Build history of the part. All positions in model axes, mm. A direction names the side the tool comes from. Give positions to 0.01 mm unless a question says otherwise; leave off trailing zeros. Order: outer loops, then holes, each group sorted by start corner. A loop starts at its lowest first (then second) coordinate and runs counter-clockwise, first axis right, second up. Notation, with made-up numbers: M 8,42.25 L 49,42.25 A10 cw 49,47.25 Z; hole C 27.25,-39.5 d7. An arc over 180 degrees is marked long. Use CSV: the item, a comma, the result in double quotes. Start each with the question number.
Item 1: Band-saw the part on C-C on x = 3.5. Write the cut outline in (y, z) (3 decimals).
Item 2: Pin check, flat tips, straight feed: P1, Ø4.5, axis at y = 14.29, z = 14.29, coming from the +X side; P2, Ø4, axis at x = 22, z = -3, coming from the +Y side; P3, Ø4, axis at x = 7.5, y = 14, coming from the -Z side. Stop position of each tip, or through.
Item 3: Band-saw the part on A-A on z = 0. Write the cut outline in (x, y) (1 decimal).
Item 4: Band-saw the part on D-D on x = 24. Write the cut outline in (y, z), plus the area to 3 significant figures.
Item 5: Two-plate mould, pull along Z, no slides. Class faces 4 (the cylindrical face through (11.845, 16.176, 14.04)), 5 (the cylindrical face through (11.85, -17.32, 17.37)), 6 (the flat face through (12, -18.224, 0)): pulls with the +Z half, pulls with the -Z half, needs draft (parallel to the pull), parting line crosses it, or undercut.
Item 6: Wall check: line 1 along X through (y, z) = (-2, 15.5); line 2 along Y through (x, z) = (20.5, -0.5); line 3 along Y through (x, z) = (16.75, 10). Give the ranges that are in metal, low to high.
Item 7: Which spindle directions (+Z, -Z, +X, -X, +Y, -Y) get a long thin tool onto all of the face, cutting with end or side? Do faces 1 (the cylindrical face through (11.85, 17.32, -17.37)), 2 (the flat face through (10.668, -12, 8)), 3 (the cylindrical face through (20.216, -4.158, 13.204)). Say none if no direction does.
from build123d import *

# Parameters (mm, degrees)
SKETCH2_OUTSIDE_W  = 79.82
SKETCH2_OUTSIDE_H  = 79.82
SKETCH2_OUTSIDE_R  = 1.905
CUT_EXTRUDE1_DEPTH = 17.51


with BuildPart() as part:
    # Sketch1 → Revolve1 (revolve)
    with BuildSketch(Plane.XY, mode=Mode.PRIVATE) as revolve1_sk:
        Polygon((0, 0), (0, 13.335), (10.668, 13.335), (10.668, 30), (13.0556, 30), (13.0556, 13.843), (27.178, 13.843), (27.178, 0), align=None)
    revolve(revolve1_sk.sketch.rotate(Axis((0, 0, 0), (1, 0, 0)), 90), axis=Axis((0, 0, 0), (1, 0, 0)))  # turned: the seam where the file's is

    # Sketch2 outside → Cut-Extrude1 (cut, through all)
    with BuildSketch(Plane.ZY.offset(-10.668)):
        Rectangle(SKETCH2_OUTSIDE_W, SKETCH2_OUTSIDE_H)
        with BuildLine():
            Line((-15.2245, 18.2245), (15.2245, 18.2245))
            ThreePointArc((15.2245, 18.2245), (17.345820344, 17.345820344), (18.2245, 15.2245))
            Line((18.2245, 15.2245), (18.2245, -15.2245))
            ThreePointArc((18.2245, -15.2245), (17.345820344, -17.345820344), (15.2245, -18.2245))
            Line((15.2245, -18.2245), (-15.2245, -18.2245))
            ThreePointArc((-15.2245, -18.2245), (-17.345820344, -17.345820344), (-18.2245, -15.2245))
            Line((-18.2245, -15.2245), (-18.2245, 15.2245))
            ThreePointArc((-18.2245, 15.2245), (-17.345820344, 17.345820344), (-15.2245, 18.2245))
        make_face(mode=Mode.SUBTRACT)
        with Locations((14.2875, 14.2875)):
            Circle(SKETCH2_OUTSIDE_R)
        with Locations((-14.2875, 14.2875)):
            Circle(SKETCH2_OUTSIDE_R)
        with Locations((-14.2875, -14.2875)):
            Circle(SKETCH2_OUTSIDE_R)
        with Locations((14.2875, -14.2875)):
            Circle(SKETCH2_OUTSIDE_R)
    extrude(amount=-CUT_EXTRUDE1_DEPTH, mode=Mode.SUBTRACT)


solid = part.part
Model answer:
1,outline,"C 0,0 d26.67"
2,P1,"stops at x = 13.06"
2,P2,"stops at y = 13.81"
2,P3,"stops at z = -5.82"
3,outline,"M 0,-13.3 L 10.7,-13.3 L 10.7,-18.2 L 13.1,-18.2 L 13.1,-13.8 L 27.2,-13.8 L 27.2,13.8 L 13.1,13.8 L 13.1,18.2 L 10.7,18.2 L 10.7,13.3 L 0,13.3 Z"
4,outline,"C 0,0 d27.69"
4,area,"602 mm^2"
5,face 4,"undercut"
5,face 5,"pulls with the +Z half"
5,face 6,"needs draft"
6,line 1,"x = 10.67 to 13.06"
6,line 2,"y = -13.83 to 13.83"
6,line 3,"y = -9.57 to 9.57"
7,face 1,"-Z, +X, -X, +Y"
7,face 2,"-X"
7,face 3,"+X"
